Can you work these out from the model? Positions are in its coordinate system, mm. Face numbers are marked on the shaded views. A direction names the side the tool comes from. Round coordinates to 2 decimals unless told otherwise and drop trailing zeros. Order: outer loops, then holes, each group sorted by start corner. A loop starts at its lowest first (then second) coordinate and runs counter-clockwise, first axis right, second up.
Q1. We'd pull the mould along Y, two halves only. Please class the marked faces 3, 4, 5 and 6: pulls with the +Y half, pulls with the -Y half, needs draft (parallel to the pull), parting line crosses it, or undercut.
Q2. If I drill on line 1 (X direction, y = -26, z = 6); line 2 (Z direction, x = 8, y = -42.5); line 3 (Z direction, x = 26, y = -23.5), over which ranges is the centre line in solid material (lowest first)?
Q3. If we section it at A-A (z = 22): Please give me the cut outline in (x, y), plus the area to 3 significant figures.
Q4. If we section it at C-C (x = 9.5): Please give me the cut outline in (y, z).
Q5. If we section it at D-D (y = -7.5): Please give me the cut outline in (x, z).
Q6. Will these pins go through, and if not, where does the flat tip stop? P1, Ø6, axis at x = -11.5, y = -16.5, coming from the +Z side; P2, Ø16.5, axis at y = -24.89, z = 17.48, coming from the -X side.
Q7. For the marked faces 1 and 2, which set-ups out of +Z, -Z, +X, -X, +Y, -Y let a thin tool reach every point of the face, with its end or its side?
Q8. If we section it at B-B (y = -26): Please give me the cut outline in (x, z), plus the area to 3 significant figures.
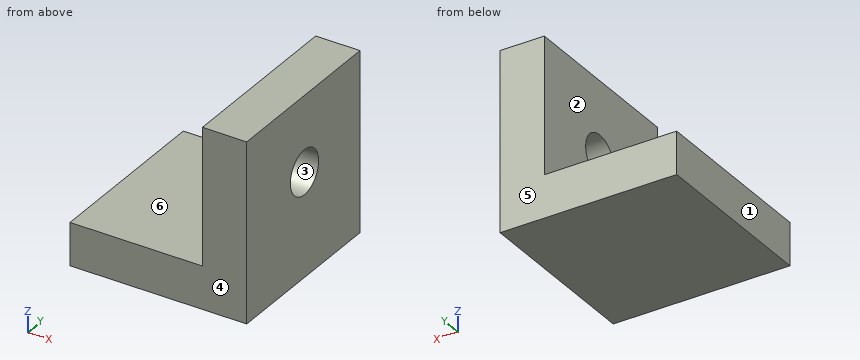
from build123d import *

# Parameters (mm, degrees)
F0_W     = 50.6729986519
F0_H     = 51.3397492468
F1_DEPTH = 50.8
F2_W     = 37.9729986519
F2_H     = 39.115998894
F5_DEPTH = 25.4
F6_DEPTH = 25.4
F7_R     = 6.35
F8_DEPTH = 25.4


with BuildPart() as f1:
    # F0 (on Front) → F1 (new body)
    with BuildSketch(Plane.XZ):
        with Locations((4.444998689, 13.4461242706)):
            Rectangle(F0_W, F0_H)
    extrude(amount=F1_DEPTH)

    # F2 (on face) → F5 (cut)
    with BuildSketch(Plane(origin=(0, 0, 0), x_dir=(-1, 0, 0), z_dir=(0, 1, 0))):
        with Locations((1.905001311, 19.557999447)):
            Rectangle(F2_W, F2_H)
    extrude(amount=-F5_DEPTH, mode=Mode.SUBTRACT)

    # F6 (cut): a face of the model
    f6_faces = [f1.faces().sort_by_distance(p)[0] for p in [
        (-1.905001311, -25.4, 19.557999447),
    ]]
    extrude(f6_faces, amount=-F6_DEPTH, mode=Mode.SUBTRACT)

    # F7 (on face) → F8 (cut)
    with BuildSketch(Plane(origin=(17.0814980149, 0, 0), x_dir=(0, -1, 0), z_dir=(-1, 0, 0))):
        with Locations((24.8914603144, 17.4777153879)):
            Circle(F7_R)
    extrude(amount=-F8_DEPTH, mode=Mode.SUBTRACT)


solid = f1.part
Solution:
1. face 3: undercut
1. face 4: pulls with the -Y half
1. face 5: pulls with the +Y half
1. face 6: needs draft
2. line 1: x = 17.08 to 29.78
2. line 2: z = -12.22 to 0
2. line 3: z = -12.22 to 11.28, 23.67 to 39.12
3. outline: (17.08, -50.8) - (29.78, -50.8) - (29.78, -29.35) - (17.08, -29.35) - close; (17.08, -20.43) - (29.78, -20.43) - (29.78, 0) - (17.08, 0) - close
3. area: 532 mm2
4. outline: (-50.8, -12.22) - (0, -12.22) - (0, 0) - (-50.8, 0) - close
5. outline: (-20.89, -12.22) - (29.78, -12.22) - (29.78, 39.12) - (17.08, 39.12) - (17.08, 0) - (-20.89, 0) - close
6. P1: stops at z = 0
6. P2: stops at x = 17.08
7. face 1: +Z, -Z, -X, +Y, -Y
7. face 2: +Z, -X, +Y, -Y
8. outline: (-20.89, -12.22) - (29.78, -12.22) - (29.78, 11.23) - (17.08, 11.23) - (17.08, 0) - (-20.89, 0) - close; (17.08, 23.73) - (29.78, 23.73) - (29.78, 39.12) - (17.08, 39.12) - close
8. area: 957 mm2
